Could you check a few things on this model? Use its own coordinates, in mm. Coordinates: 2 decimals unless noted, no trailing zeros. Order: outer loops, then holes, each group sorted by start corner. A loop starts at its lowest first (then second) coordinate and runs counter-clockwise, first axis right, second up. Notation, with made-up numbers: (19.25, 66) - (54.25, 66) arc R15 ccw to (54.25, 90) - close; hole circle Ø2 at (60.5, -25). An arc over 180 degrees is marked (long way). Answer as a JSON object with one key per item and string values. Group by question number.
(1) Will these pins go through, and if not, where does the flat tip stop? P1, Ø8, axis at x = -14.5, y = -409, coming from the -Z side; P2, Ø6, axis at x = -9.5, z = 18, coming from the -Y side; P3, Ø8, axis at y = -198.5, z = 15, coming from the -X side.
(2) Imagine slicing it at B-B, the plane y = -463. Write out the boundary of the cut face in (x, z).
(3) Imagine slicing it at A-A, the plane y = -20. Write out the boundary of the cut face in (x, z).
(4) Please list where these lines run through material, in increasing order: probe 1 along Y at (x, z) = (-10.5, 3); probe 2 along X at (y, z) = (-268.5, 2); probe 3 along Y at (x, z) = (-13.5, 15).
from build123d import *

# Parameters (mm, degrees)
F0_R      = 25
F0_R_2    = 20
F1_DEPTH  = 500
F2_R      = 25
F3_DEPTH  = 5
F5_DEPTH  = 20
F7_D      = 5
F10_D     = 12
F10_DEPTH = 6
F10_START = 0.7306779
F10_TIP   = 3.6051637142
F12_DEPTH = 20
F17_D     = 12
F17_DEPTH = 6
F17_START = 0.7306779
F17_TIP   = 3.6051637142
F19_D     = 12
F19_DEPTH = 6
F19_START = 0.7306779
F19_TIP   = 3.6051637142
F20_R     = 5
F22_R     = 25
F22_R_2   = 24
F23_DEPTH = 1
F25_R     = 25
F25_R_2   = 24
F26_DEPTH = 1


with BuildPart() as f1:
    # F0 (on Front) → F1 (new body)
    with BuildSketch(Plane.XZ):
        Circle(F0_R)
        Circle(F0_R_2, mode=Mode.SUBTRACT)
    extrude(amount=F1_DEPTH)

    # F2 (on face) → F3 (join)
    with BuildSketch(Plane.XZ.offset(500)):
        Circle(F2_R)
    extrude(amount=F3_DEPTH)

    # F4 (on face) → F5 (join)
    with BuildSketch(Plane.XZ.offset(505)):
        Polygon((-16.0628025015, -5.6190539991), (0.380358971, -17.013016167), (16.2978772735, -4.8955682433), (9.6922831285, 13.9873885984), (-10.3077168715, 13.540249811), align=None)
    extrude(amount=F5_DEPTH)

    # F7 (through all)
    with Locations(Plane.XZ.offset(525)):
        with Locations((0, 0)):
            Hole(F7_D / 2)

    # F10
    # its depths count from where the whole tool has entered the part; down to there all is cleared
    with Locations(Plane.YZ.offset(25).offset(-F10_START)):
        with Locations((-20, 0), (-130, 0)):
            Hole(F10_D / 2, depth=F10_DEPTH)
            with Locations((0, 0, -(F10_DEPTH + F10_TIP / 2))):  # 118° drill point
                Cone(0, F10_D / 2, F10_TIP, mode=Mode.SUBTRACT)

    # F11 (on face) → F12 (join)
    with BuildSketch(Plane(origin=(0, 0, 0), x_dir=(-1, 0, 0), z_dir=(0, 1, 0))):
        Polygon((12.5, -21.6506350946), (12.5, 21.6506350946), (-25, 0), align=None)
    extrude(amount=F12_DEPTH)

    # F17
    # its depths count from where the whole tool has entered the part; down to there all is cleared
    with Locations(Plane(origin=(-12.5, 0, -21.6506350946), x_dir=(0.8660254038, 0, -0.5), z_dir=(-0.5, 0, -0.8660254038)).offset(-F17_START)):
        with Locations((0, 20), (0, 130)):
            Hole(F17_D / 2, depth=F17_DEPTH)
            with Locations((0, 0, -(F17_DEPTH + F17_TIP / 2))):  # 118° drill point
                Cone(0, F17_D / 2, F17_TIP, mode=Mode.SUBTRACT)

    # F19
    # its depths count from where the whole tool has entered the part; down to there all is cleared
    with Locations(Plane(origin=(-12.5, 0, 21.6506350946), x_dir=(0.8660254038, 0, 0.5), z_dir=(-0.5, 0, 0.8660254038)).offset(-F19_START)):
        with Locations((0, -20), (0, -130)):
            Hole(F19_D / 2, depth=F19_DEPTH)
            with Locations((0, 0, -(F19_DEPTH + F19_TIP / 2))):  # 118° drill point
                Cone(0, F19_D / 2, F19_TIP, mode=Mode.SUBTRACT)

    # F20
    f20_edges = [f1.edges().sort_by_distance(p)[0] for p in [
        (6.25, 20, 10.825318),
        (-12.5, 20, 0),
        (6.25, 20, -10.825318),
    ]]
    fillet(f20_edges, radius=F20_R)

    # F22 (on offset) → F23 (cut)
    with BuildSketch(Plane.XZ.offset(250)):
        Circle(F22_R)
        Circle(F22_R_2, mode=Mode.SUBTRACT)
    extrude(amount=-F23_DEPTH, mode=Mode.SUBTRACT)

    # F25 (on offset) → F26 (cut)
    with BuildSketch(Plane.XZ.offset(350)):
        Circle(F25_R)
        Circle(F25_R_2, mode=Mode.SUBTRACT)
    extrude(amount=F26_DEPTH, mode=Mode.SUBTRACT)


solid = f1.part
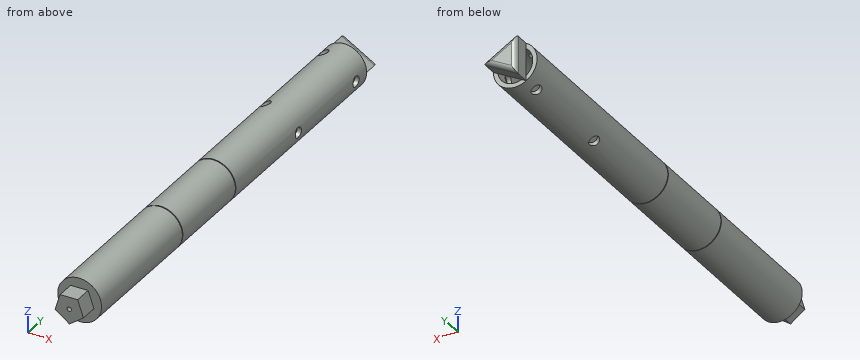
Result set:
{
 "1": {"P1": "stops at z = -22.69", "P2": "stops at y = -505", "P3": "stops at x = -22.45"},
 "2": {"outline": "circle Ø50 at (0, 0); hole circle Ø40 at (0, 0)"},
 "3": {"outline": "(-17.33, -18.02) - (-14.74, -13.52) arc R20 cw to (-14.74, 13.52) - (-17.33, 18.02) arc R25 ccw to start; (-6.94, -24.02) arc R25 ccw to (24.27, -6) - (19.08, -6) arc R20 cw to (-4.34, -19.52) - close; (-6.94, 24.02) - (-4.34, 19.52) arc R20 cw to (19.08, 6) - (24.27, 6) arc R25 ccw to start"},
 "4": {"probe 1": "y = -525 to -500, 0 to 19", "probe 2": "x = -24.92 to -19.9, 19.9 to 24.92", "probe 3": "y = -505 to -134.29, -125.71 to -24.29, -15.71 to 0"}
}
